For this review, use the dimensioned drawing (mm, ordinates from the lowest corner) and the shaded views. A direction names the side the tool comes from. Round coordinates to 2 decimals unless told otherwise and drop trailing zeros. Write each loop counter-clockwise with the first axis right and the second up, starting at its lowest first coordinate (ties: lowest second). Pieces come first, ordered by that corner, then holes.
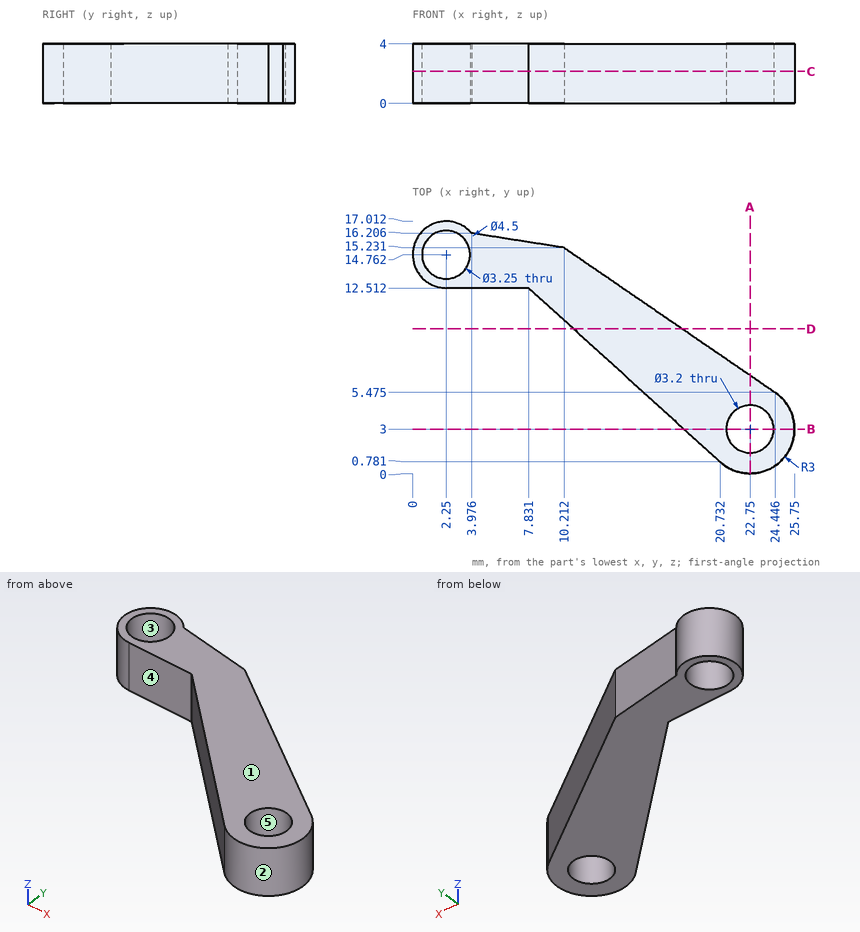
1) Add section B-B on y = 3. State the section outline as (x, z) points.
2) Add section C-C on z = 2.15. Count the separate pieces of the cut face and the enclosed holes in it, and give its area (3 significant figures).
3) For P1, Ø1.2, axis at x = 4.5, z = 1.5, coming from the -Y side; P2, Ø1.5, axis at x = 13.5, z = 3, coming from the -Y side (1 decimal); P3, Ø2, axis at y = 4.5, z = 0.5, coming from the -X side, all flat-tipped, find the tip position at first contact; note any pin that passes through.
4) For line 1 along Y through (x, z) = (2.25, 1.15); line 2 along X through (y, z) = (14.75, 0.2) (1 decimal); line 3 along X through (y, z) = (2.25, 2.4) (1 decimal), list the stretches that pass through material, from the lowest coordinate up.
5) For the marked faces 4 and 5, list the 3-axis set-ups (+Z, -Z, +X, -X, +Y, -Y) from which the entire face can be reached by the end or side of a thin tool; tool diameter is ignored.
6) Add section A-A on x = 22.75. State the section outline as (y, z) points.
7) The part is to be moulded in two halves that separate along Y. For the marked faces 1, 2 and 3, say which applies: pulls with the +Y half, pulls with the -Y half, needs draft (parallel to the pull), parting line crosses it, or undercut.
8) Add section D-D on y = 9.75. State the section outline as (x, z) points.
Computed:
1. outline: (18.29, 0) - (21.15, 0) - (21.15, 4) - (18.29, 4) - close; (24.35, 0) - (25.75, 0) - (25.75, 4) - (24.35, 4) - close
2. separate pieces: 1
2. enclosed holes: 2
2. area: 114 mm2
3. P1: stops at y = 12.51
3. P2: stops at y = 6.7
3. P3: stops at x = 15.54
4. line 1: y = 12.51 to 13.14, 16.39 to 17.01
4. line 2: x = 0 to 0.6, 3.9 to 10.9
4. line 3: x = 19.1 to 21.3, 24.2 to 25.7
5. face 4: +Z, -Z, -X, -Y
5. face 5: +Z, -Z
6. outline: (0, 0) - (1.4, 0) - (1.4, 4) - (0, 4) - close; (4.6, 0) - (6.64, 0) - (6.64, 4) - (4.6, 4) - close
7. face 1: needs draft
7. face 2: parting line crosses it
7. face 3: undercut
8. outline: (10.87, 0) - (18.21, 0) - (18.21, 4) - (10.87, 4) - close
